from build123d import *

# Parameters (mm, degrees)
SKETCH1_R           = 75
BOSS_EXTRUDE1_DEPTH = 50
SHELL1_T            = 2.4
SKETCH2_R           = 21
SKETCH2_R_2         = 1.75
CUT_EXTRUDE1_DEPTH  = 121.3391873
BOSS_EXTRUDE3_START = -2.4
BOSS_EXTRUDE3_DEPTH = 2.4
FILLET1_R           = 2.4
SKETCH5_R           = 10
BOSS_EXTRUDE5_DEPTH = 12.4
SKETCH6_R           = 4.7
SKETCH6_R_2         = 2.2
CUT_EXTRUDE2_DEPTH  = 132.12879182


with BuildPart() as part:
    # Sketch1 → Boss-Extrude1 (new body)
    with BuildSketch(Plane(origin=(0, 0, 0), x_dir=(1, 0, 0), z_dir=(0, 1, 0))):
        with Locations(Location((0, 0, 0), (0, 0, 270))):
            Circle(SKETCH1_R)
    extrude(amount=BOSS_EXTRUDE1_DEPTH)

    # Shell1
    shell1_openings = [part.faces().sort_by_distance(p)[0] for p in [
        (0, 50, 0),
    ]]
    offset(amount=SHELL1_T, openings=shell1_openings, kind=Kind.INTERSECTION)

    # Sketch2 → Cut-Extrude1 (cut, through all)
    with BuildSketch(Plane(origin=(0, 0, 0), x_dir=(1, 0, 0), z_dir=(0, 1, 0))):
        with Locations(Location((0, -54, 0), (0, 0, 270))):
            Circle(SKETCH2_R)
        with Locations(Location((0, -27.5, 0), (0, 0, 270))):
            Circle(SKETCH2_R_2)
        with Locations(Location((22.9496732, -67.25, 0), (0, 0, 270))):
            Circle(SKETCH2_R_2)
        with Locations(Location((-22.9496732, -67.25, 0), (0, 0, 270))):
            Circle(SKETCH2_R_2)
    extrude(amount=-CUT_EXTRUDE1_DEPTH, mode=Mode.SUBTRACT)

    # Sketch3 → Boss-Extrude3 (add)
    with BuildSketch(Plane(origin=(0, 0, 0), x_dir=(1, 0, 0), z_dir=(0, 1, 0)).offset(BOSS_EXTRUDE3_START)):
        with BuildLine():
            ThreePointArc((-24.888501361, -70.75), (0, -84), (24.888501361, -70.75))
            ThreePointArc((24.888501361, -70.75), (0, -75), (-24.888501361, -70.75))
        make_face()
    extrude(amount=BOSS_EXTRUDE3_DEPTH)

    # Fillet1
    fillet1_edges = [part.edges().sort_by_distance(p)[0] for p in [
        (-22.237685481, -1.2, 74.136666667),
        (22.237685481, -1.2, 74.136666667),
        (11.237926855, 0, 76.579821102),
    ]]
    fillet(fillet1_edges, radius=FILLET1_R)

    # Sketch5 → Boss-Extrude5 (add)
    with BuildSketch(Plane(origin=(75, 0, 0), x_dir=(0, 0, -1), z_dir=(1, 0, 0))):
        with Locations(Location((0, 7.6, 0), (0, 0, 270))):
            Circle(SKETCH5_R)
    boss_extrude5 = extrude(amount=BOSS_EXTRUDE5_DEPTH)

    # Mirror1: Boss-Extrude5 across plane
    add(boss_extrude5.mirror(Plane(origin=(0, 0, 0), x_dir=(0, 0, 1), z_dir=(1, 0, 0))))

    # Sketch6 → Cut-Extrude2 (cut, through all)
    with BuildSketch(Plane(origin=(0, 0, 0), x_dir=(1, 0, 0), z_dir=(0, 1, 0))):
        with Locations(Location((0, 0, 0), (0, 0, 270))):
            Circle(SKETCH6_R)
        with Locations(Location((17.5, 8, 0), (0, 0, 270))):
            Circle(SKETCH6_R_2)
        with Locations(Location((-17.5, 8, 0), (0, 0, 90))):
            Circle(SKETCH6_R_2)
    extrude(amount=-CUT_EXTRUDE2_DEPTH, mode=Mode.SUBTRACT)


solid = part.part
The listing builds one solid part. Answer for the finished solid, in the listing's coordinates (mm). A direction names the side the tool comes from. Give positions to 0.01 mm unless a question says otherwise; leave off trailing zeros. Loops run counter-clockwise (first coordinate to the right, second up) from the corner with the lowest first, then second, coordinate; pieces in that order, holes last. Notation, with made-up numbers: (-27, 51.25) - (30, 51.25) arc R6 cw to (30, 55.25) - close; hole circle Ø3 at (19.25, -17.5). An arc over 180 degrees is marked (long way). Answer as a JSON object with one key per item and string values.
1. A cutting plane is placed at D-D (x = 32.5). Write down the section's boundary in (y, z).
Determined:
{"outline": "(-2.4, -70.25) - (50, -70.25) - (50, -67.59) - (0, -67.59) - (0, 67.59) - (50, 67.59) - (50, 70.25) - (-2.4, 70.25) - close"}
2. A cutting plane is placed at A-A (y = 7.6). Write down the section's boundary in (x, z).
Determined:
{"outline": "(-87.4, -10) - (-76.75, -10) arc R77.4 ccw to (76.75, -10) - (87.4, -10) - (87.4, 10) - (76.75, 10) arc R77.4 ccw to (-76.75, 10) - (-87.4, 10) - close; hole circle Ø150 at (0, 0)"}
3. Find the intervals of material crossed by L1, parallel to Z at x = -0.5, y = 9; L2, parallel to X at y = -1, z = 0; L3, parallel to X at y = -1, z = 67, in increasing order. Write a range as [from, to].
Determined:
{"L1": "[-77.4, -75], [75, 77.4]", "L2": "[-87.4, -4.7], [4.7, 87.4]", "L3": "[-38.75, -24.68], [-21.22, -16.49], [16.49, 21.22], [24.68, 38.75]"}
4. For faces 1 (the flat face through (1, 0, -18)), 2 (the flat face through (1, -2.4, -16)), 3 (the cylindrical face through (82, 17.59, -0.44)), determine the directions among +Z, -Z, +X, -X, +Y, -Y from which every point of the face is accessible in a straight line to the end or side of a thin tool.
Determined:
{"face 1": "+Y", "face 2": "+Z, -Z, +X, -X, -Y", "face 3": "+X"}
5. For a pull along Z with two mould halves and no side action, classify faces 4 (the cylindrical face through (0, -1, 84)), 5 (the cylindrical face through (0.92, -1.18, 33.02)), 6 (the flat face through (87.4, 8, 0)), 7 (the cylindrical face through (-82, 17.59, -0.44)) as pulls with the +Z half, pulls with the -Z half, needs draft (parallel to the pull), parting line crosses it, or undercut.
Determined:
{"face 4": "pulls with the +Z half", "face 5": "undercut", "face 6": "needs draft", "face 7": "parting line crosses it"}
6. A cutting plane is placed at B-B (z = 54). Write down the section's boundary in (x, y).
Determined:
{"outline": "(-55.45, -2.4) - (-21, -2.4) - (-21, 0) - (-52.05, 0) - (-52.05, 50) - (-55.45, 50) - close; (21, -2.4) - (55.45, -2.4) - (55.45, 50) - (52.05, 50) - (52.05, 0) - (21, 0) - close"}
7. A cutting plane is placed at C-C (z = -8). Write down the section's boundary in (x, y), then the cut area to 3 significant figures.
Determined:
{"outline": "(-87.4, 1.6) - (-76.99, 1.6) - (-76.99, -2.4) - (-19.7, -2.4) - (-19.7, 0) - (-74.57, 0) - (-74.57, 50) - (-76.99, 50) - (-76.99, 13.6) - (-87.4, 13.6) - close; (-15.3, -2.4) - (15.3, -2.4) - (15.3, 0) - (-15.3, 0) - close; (19.7, -2.4) - (76.99, -2.4) - (76.99, 1.6) - (87.4, 1.6) - (87.4, 13.6) - (76.99, 13.6) - (76.99, 50) - (74.57, 50) - (74.57, 0) - (19.7, 0) - close", "area": "840 mm²"}
8. Flat-ended cylindrical pins translate along their axes: pin 1 Ø1.9 at (x, z) = (0, 81) entering from +Y; pin 2 Ø5 at (y, z) = (17, -25) entering from +X; pin 3 Ø8 at (x, y) = (21.5, 28) entering from -Z. Find the tip coordinate at first contact, or state that the pin passes through.
Determined:
{"pin 1": "y = 0", "pin 2": "x = 74.06", "pin 3": "z = -75.4"}
